Check sheet for the modelled part. Datum: model origin and axes. Units: mm. Face numbers are marked on the shaded views. A direction names the side the tool comes from. Round coordinates to 2 decimals unless told otherwise and drop trailing zeros. Write each loop counter-clockwise with the first axis right and the second up, starting at its lowest first coordinate (ties: lowest second). Pieces come first, ordered by that corner, then holes. Notation, with made-up numbers: (83, -22.75) -> (136, -22.75) arc R19 ccw to (136, 12.25) -> close; hole circle Ø2 at (-15.75, 84.5). An arc over 180 degrees is marked (long way). Use one line per item in the form item = value. Start each with the question number.
Autodesk Inventor part; units mm, degrees
ref_plane "YZ Plane" through (0, 0, 0) normal (1, 0, 0) x (0, 1, 0)
ref_plane "XZ Plane" through (0, 0, 0) normal (0, 1, 0) x (-1, 0, 0)
ref_plane "XY Plane" through (0, 0, 0) normal (0, 0, 1) x (1, 0, 0)
sketch "Sketch1" plane through (0, 0, 0) normal (0, 1, 0) x (-1, 0, 0)
  line L0 (0, 0) -> (38.1, 0)
  line L1 (38.1, 0) -> (38.1, -101.6)
  line L2 (38.1, -101.6) -> (0, -101.6)
  line L3 (0, -101.6) -> (0, 0)
  line L4 (38.1, -101.6) -> (33.02, -101.6)
  line L5 (33.02, -101.6) -> (33.02, 0)
  line L6 (33.02, 0) -> (38.1, 0)
  line L7 (38.1, 0) -> (38.1, -101.6)
  line L8 (0, -101.6) -> (5.08, -101.6)
  line L9 (5.08, -101.6) -> (5.08, 0)
  line L10 (5.08, 0) -> (0, 0)
  line L11 (0, 0) -> (0, -101.6)
  dimension "d0" = 38.1
  dimension "d1" = 101.6
  dimension "d2" = 5.08
  dimension "d3" = 5.08
extrude "Extrusion1" add sketch "Sketch1" along normal blind 25.4 contours L0 L9 L2 L3 | L0 L1 L2 L5
extrude "Extrusion2" add sketch "Sketch1" against normal blind 5.08
sketch "Sketch2" plane through (0, 25.4, 0) normal (1, 0, 0) x (0, 0, -1)
  line L0 (101.6, 0) -> (0, 0)
  line L1 (50.8, 0) -> (50.8, -12.7)
  point P0 (0, -25.4)
  dimension "d8" = 12.7
hole "Hole1" at (0, 12.7, -50.8) direction (-1, 0, 0) diameter 6.7564 end through all
sketch "Sketch3" plane through (0, -5.08, 0) normal (0, -1, 0) x (1, 0, 0)
  line L0 (0, -101.6) -> (-5.08, -101.6)
  line L1 (0, -101.6) -> (0, -88.9)
  line L2 (0, 0) -> (0, -101.6)
  line L3 (0, -88.9) -> (0, -63.5)
  line L4 (0, -88.9) -> (-19.05, -88.9)
  line L5 (0, -63.5) -> (-19.05, -63.5)
  line L6 (-38.1, -101.6) -> (-38.1, 0)
  line L7 (0, -90.4875) -> (-38.1, -90.4875)
  line L8 (-38.1, -90.4875) -> (-38.1, -87.3125)
  line L9 (-38.1, -87.3125) -> (0, -87.3125)
  line L10 (0, -87.3125) -> (0, -90.4875)
  line L11 (0, -90.4875) -> (-38.1, -87.3125) construction
  line L12 (-38.1, -90.4875) -> (0, -87.3125) construction
  line L13 (0, -61.9125) -> (-38.1, -61.9125)
  line L14 (-38.1, -61.9125) -> (-38.1, -65.0875)
  line L15 (-38.1, -65.0875) -> (0, -65.0875)
  line L16 (0, -65.0875) -> (0, -61.9125)
  line L17 (0, -61.9125) -> (-38.1, -65.0875) construction
  line L18 (-38.1, -61.9125) -> (0, -65.0875) construction
  line L19 (-38.1, 0) -> (-38.1, -101.6)
  line L20 (-38.1, 0) -> (0, 0)
  line L21 (0, 0) -> (0, -3.175)
  line L22 (0, -3.175) -> (-38.1, -3.175)
  line L23 (-38.1, -3.175) -> (-38.1, 0)
  line L24 (0, -101.6) -> (-38.1, -101.6)
  line L25 (-38.1, -101.6) -> (-38.1, -98.425)
  line L26 (-38.1, -98.425) -> (0, -98.425)
  line L27 (0, -98.425) -> (0, -101.6)
  line L28 (0, -3.175) -> (0, -28.575)
  line L29 (-38.1, -98.425) -> (-38.1, -73.025)
  line L30 (-38.1, -98.425) -> (-12.7, -98.425) construction
  line L31 (0, -28.575) -> (-38.1, -28.575)
  line L32 (-38.1, -28.575) -> (-38.1, -31.115)
  line L33 (-38.1, -31.115) -> (0, -31.115)
  line L34 (0, -31.115) -> (0, -28.575)
  line L35 (-38.1, -73.025) -> (0.7144, -73.025)
  line L36 (0.7144, -73.025) -> (0.7144, -70.485)
  line L37 (0.7144, -70.485) -> (-38.1, -70.485)
  line L38 (-38.1, -70.485) -> (-38.1, -73.025)
  point P0 (0, -65.0875)
  point P1 (0, -61.9125)
  point P2 (0, -87.3125)
  point P3 (-38.1, -90.4875)
  point P4 (0, -90.4875)
  point P5 (0, -98.425)
  point P6 (-38.1, -98.425)
  point P7 (0, -31.115)
  dimension "d16" = 12.7
  dimension "d17" = 25.4
  dimension "d18" = 19.05
  dimension "d19" = 3.175
  dimension "d20" = 3.175
  dimension "d32" = 3.175
  dimension "d33" = 3.175
  dimension "d34" = 25.4
  dimension "d35" = 25.4
  dimension "d36" = 90
  dimension "d37" = 2.54
  dimension "d38" = 2.54
extrude "Extrusion3" add sketch "Sketch3" along normal blind 25.4 contours L0 L24 L6 L26 L1 | L35 L6 L37 L2 | L2 L37 L36 L35 | L6 L31 L2 L33 | L6 L20 L2 L22
sketch "Sketch4" plane through (-38.1, -5.08, 0) normal (0, 0, 1) x (1, 0, 0)
  line L0 (38.1, -25.4) -> (19.05, -25.4)
  line L1 (19.05, -25.4) -> (19.05, -13.97)
  point P0 (38.1, 5.08)
  dimension "d23" = 11.43
hole "Hole2" at (-19.05, -19.05, 0) direction (0, 0, -1) diameter 2.8575 end through all
sketch "Sketch5" plane through (0, -30.48, 0) normal (0, -1, 0) x (1, 0, 0)
  line L0 (-38.1, -3.175) -> (-38.1, -28.575)
  line L1 (0, 0) -> (-38.1, 0)
  line L2 (-38.1, 0) -> (-38.1, -3.175)
  line L3 (-38.1, -3.175) -> (0, -3.175)
  line L4 (0, -3.175) -> (0, 0)
  line L5 (-38.1, -101.6) -> (-38.1, 0)
  line L6 (0, 0) -> (0, -101.6)
  line L7 (-38.1, -101.6) -> (0, -101.6)
  line L8 (0, -101.6) -> (0, -98.4864)
  line L9 (0, -98.4864) -> (-38.1, -98.4864)
  line L10 (-38.1, -98.4864) -> (-38.1, -101.6)
extrude "Extrusion4" add sketch "Sketch5" along normal blind 101.6 contours L2 L1 L4 L3 | L9 L6 L7 L5
sketch "Sketch6" plane through (-38.1, -30.48, -98.4864) normal (0, 0, 1) x (1, 0, 0)
  line L0 (0, 55.88) -> (0, -101.6)
  line L1 (38.1, 0) -> (38.1, -101.6)
  line L2 (0, -101.6) -> (38.1, -101.6)
  line L3 (38.1, -101.6) -> (38.1, -96.52)
  line L4 (38.1, -96.52) -> (0, -96.52)
  line L5 (0, -96.52) -> (0, -101.6)
  point P0 (38.1, 30.48)
  dimension "d41" = 5.08
extrude "Extrusion5" add sketch "Sketch6" along normal blind 96.52
properties part number "Sample Holder end for 8020-thruhole-widestance-long-withoverheadcam"
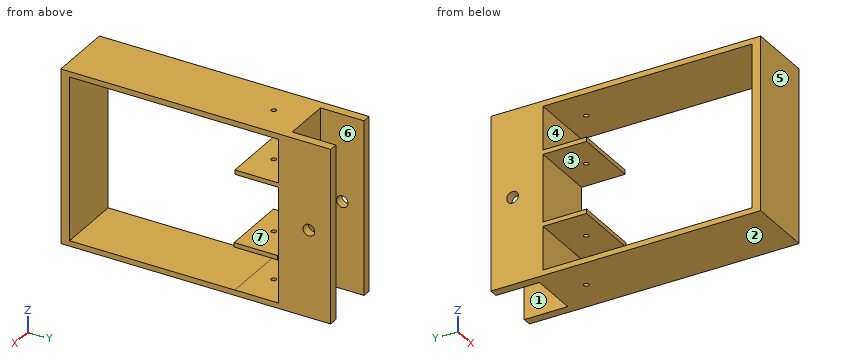
1. Scan lines: probe 1 along Z at (x, y) = (-9.5, -9) (3 decimals); probe 2 along Y at (x, z) = (-19, -72); probe 3 along Z at (x, y) = (-1.75, 12.7). Record each from-to range of solid material in increasing order.
2. Sectioned sample at B-B (z = -50.8). Enter the section's corners in (x, y).
3. Mould release check, pull along Y, two halves, no side actions. Record for the marked faces 4, 5, 6 and 7: +Y half, -Y half, draft (parallel to the pull), parting line (faces both ways), or undercut.
4. Tool access check on the marked faces 1, 2 and 3. Record the directions out of +Z, -Z, +X, -X, +Y, -Y that give a thin tool (end or side, any length) a straight path to the whole face; none if there is none.
5. Depth check by flat-ended pin: pin 1 (0.8 mm diameter, centred on x = 0.5, z = -72, fed in from +Y); pin 2 (1.7 mm diameter, centred on x = -19.05, y = -19.05, fed in from +Z); pin 3 (11.5 mm diameter, centred on x = -13.5, z = -55.5, fed in from +Y). Enter the tip coordinate at first touch or a pass-through.
6. Sectioned sample at A-A (y = -86). Enter the section's corners in (x, z) (3 decimals).
7. Sectioned sample at D-D (y = 12.7). Enter the section's corners in (x, z), and give its area (3 significant figures).
8. Sectioned sample at C-C (x = -2.5). Enter the section's corners in (y, z) (3 decimals).
Returned:
q1.probe_1 = -101.6 to -98.425, -73.025 to -70.485, -31.115 to -28.575, -3.175 to 0
q1.probe_2 = -132.08 to -127, -30.48 to -20.48, -17.62 to 0
q1.probe_3 = -101.6 to -54.18, -47.42 to 0
q2.outline = (-38.1, -132.08) -> (0, -132.08) -> (0, -127) -> (-38.1, -127) -> close; (-38.1, -5.08) -> (0, -5.08) -> (0, 9.32) -> (-5.08, 9.32) -> (-5.08, 0) -> (-33.02, 0) -> (-33.02, 9.32) -> (-38.1, 9.32) -> close; (-38.1, 16.08) -> (-33.02, 16.08) -> (-33.02, 25.4) -> (-38.1, 25.4) -> close; (-5.08, 16.08) -> (0, 16.08) -> (0, 25.4) -> (-5.08, 25.4) -> close
q3.face_4 = undercut
q3.face_5 = -Y half
q3.face_6 = draft
q3.face_7 = undercut
q4.face_1 = +Z, -Z, +Y
q4.face_2 = -Z, +X, -X, +Y, -Y
q4.face_3 = +X, -X
q5.pin_1 = -5.08
q5.pin_2 = through
q5.pin_3 = 0
q6.outline = (-38.1, -101.6) -> (0, -101.6) -> (0, -98.486) -> (-38.1, -98.486) -> close; (-38.1, -3.175) -> (0, -3.175) -> (0, 0) -> (-38.1, 0) -> close
q7.outline = (-38.1, -101.6) -> (-33.02, -101.6) -> (-33.02, -54.18) -> (-38.1, -54.18) -> close; (-38.1, -47.42) -> (-33.02, -47.42) -> (-33.02, 0) -> (-38.1, 0) -> close; (-5.08, -101.6) -> (0, -101.6) -> (0, -54.18) -> (-5.08, -54.18) -> close; (-5.08, -47.42) -> (0, -47.42) -> (0, 0) -> (-5.08, 0) -> close
q7.area = 964 mm^2
q8.outline = (-132.08, -101.6) -> (25.4, -101.6) -> (25.4, 0) -> (-132.08, 0) -> close; hole (-127, -98.486) -> (-30.48, -98.486) -> (-30.48, -98.425) -> (-5.08, -98.425) -> (-5.08, -73.025) -> (-30.48, -73.025) -> (-30.48, -70.485) -> (-5.08, -70.485) -> (-5.08, -31.115) -> (-30.48, -31.115) -> (-30.48, -28.575) -> (-5.08, -28.575) -> (-5.08, -3.175) -> (-127, -3.175) -> close; hole circle Ø6.756 at (12.7, -50.8)
